```python
from build123d import *

# Parameters (mm, degrees)
BOSS_EXTRUDE1_DEPTH = 1.445
SKETCH2_R           = 3.2
CUT_EXTRUDE1_DEPTH  = 1.67
SKETCH3_R           = 3.2
BOSS_EXTRUDE2_DEPTH = 3.4
CUT_EXTRUDE3_DEPTH  = 36.101138158
SKETCH6_R           = 1.65
CUT_EXTRUDE4_DEPTH  = 34.904858059
BOSS_EXTRUDE3_DEPTH = 2.89
BOSS_EXTRUDE4_DEPTH = 31
BOSS_EXTRUDE5_DEPTH = 2.75
FILLET2_R           = 1


with BuildPart() as part:
    # Sketch1 → Boss-Extrude1 (new, symmetric)
    with BuildSketch(Plane.XY):
        with BuildLine():
            Line((4.65938028, -4.314241), (22.15938028, 14.585759))
            ThreePointArc((22.15938028, 14.585759), (21.814241, 23.55938028), (12.84061972, 23.214241))
            Line((12.84061972, 23.214241), (-4.65938028, 4.314241))
            ThreePointArc((-4.65938028, 4.314241), (-4.314241, -4.65938028), (4.65938028, -4.314241))
        make_face()
    extrude(amount=BOSS_EXTRUDE1_DEPTH, both=True)

    # Sketch2 → Cut-Extrude1 (cut)
    with BuildSketch(Plane.XY.offset(1.445)):
        Circle(SKETCH2_R)
        with Locations((17.5, 18.9)):
            Circle(SKETCH2_R)
    extrude(amount=-CUT_EXTRUDE1_DEPTH, mode=Mode.SUBTRACT)

    # Sketch3 → Boss-Extrude2 (add)
    with BuildSketch(Plane.XY.offset(-0.225)):
        Circle(SKETCH3_R)
        with Locations((17.5, 18.9)):
            Circle(SKETCH3_R)
    extrude(amount=-BOSS_EXTRUDE2_DEPTH)

    # Sketch5 → Cut-Extrude3 (cut, through all)
    with BuildSketch(Plane.XY.offset(1.445)):
        with BuildLine():
            Line((22.37, 14.825003067), (22.37, 22.974996933))
            ThreePointArc((22.37, 22.974996933), (23.85, 18.9), (22.37, 14.825003067))
        make_face()
    extrude(amount=-CUT_EXTRUDE3_DEPTH, mode=Mode.SUBTRACT)

    # Sketch6 → Cut-Extrude4 (cut, through all)
    with BuildSketch(Plane.XY.offset(-0.225)):
        Circle(SKETCH6_R)
        with Locations((17.5, 18.9)):
            Circle(SKETCH6_R)
    extrude(amount=-CUT_EXTRUDE4_DEPTH, mode=Mode.SUBTRACT)

    # Sketch7 → Boss-Extrude3 (add)
    with BuildSketch(Plane.XY.offset(1.445)):
        with BuildLine():
            Line((-4.65938028, 4.314241), (-13, 4.314241))
            Line((-13, 4.314241), (-13, -6.35))
            Line((-13, -6.35), (0, -6.35))
            ThreePointArc((0, -6.35), (-5.818845691, -2.542348289), (-4.65938028, 4.314241))
        make_face()
    extrude(amount=-BOSS_EXTRUDE3_DEPTH)

    # Sketch8 → Boss-Extrude4 (add)
    with BuildSketch(Plane.XZ.offset(6.35)):
        with BuildLine():
            Line((-13.837814719, 2.538922528), (-13, 1.445))
            Line((-13, 1.445), (-10.25, 1.445))
            Line((-10.25, 1.445), (-10.25, 3.755))
            ThreePointArc((-10.25, 3.755), (-12.892016574, 5.649152771), (-13.837814719, 2.538922528))
        make_face()
        Polygon((-11.25, 3.177649731), (-12.25, 2.600299462), (-13.25, 3.177649731), (-13.25, 4.332350269), (-12.25, 4.909700538), (-11.25, 4.332350269), align=None, mode=Mode.SUBTRACT)
    extrude(amount=-BOSS_EXTRUDE4_DEPTH)

    # Sketch10 → Boss-Extrude5 (add)
    with BuildSketch(Plane.ZY.offset(13)):
        Polygon((-1.445, 4.314241), (1.445, 24.65), (1.445, 4.314241), align=None)
    extrude(amount=-BOSS_EXTRUDE5_DEPTH)

    # Fillet2
    fillet2_edges = [part.edges().sort_by_distance(p)[0] for p in [
        (-4.65938028, 4.314241, 0),
        (-11.625, 24.65, 1.445),
    ]]
    fillet(fillet2_edges, radius=FILLET2_R)


solid = part.part
```
Can you work these out from the model? Positions are in its coordinate system, mm. A direction names the side the tool comes from. Give positions to 0.01 mm unless a question says otherwise; leave off trailing zeros. Order: outer loops, then holes, each group sorted by start corner. A loop starts at its lowest first (then second) coordinate and runs counter-clockwise, first axis right, second up. Notation, with made-up numbers: (70, 87.5) - (117, 87.5) arc R34 ccw to (117, 123.5) - close; hole circle Ø8 at (75, 42.25). An arc over 180 degrees is marked (long way). Use a Markdown table: item, result. Add a question column.
Q1. I'm going to push flat-ended pins straight in: pin 1 (16 mm diameter, centred on x = 2, y = 11.5, fed in from -Z) (3 decimals); pin 2 (4 mm diameter, centred on x = 16, z = 1, fed in from -Y); pin 3 (1 mm diameter, centred on x = 13.5, y = 14, fed in from +Z) (3 decimals). Where does each tip first touch, or does it pass through?
Q2. On a 3-axis mill with a long thin cutter (end or side, diameter ignored), from which of +Z, -Z, +X, -X, +Y, -Y can I reach the whole of each face in a straight line? I mean faces 1 (the flat face through (-11.743, 8.933, 2.893)), 2 (the cylindrical face through (-11.55, 24.4, 1.65)), 3 (the flat face through (-8, 4.314, 0)), 4 (the cylindrical face through (16.806, 15.776, 0.622)), 5 (the flat face through (-10.25, 9, 2)). Say none if no direction works.
Q3. Please list where these lines run through material, in increasing order: line 1 along Y through (x, z) = (0, -3); line 2 along Y through (x, z) = (-9, 0); line 3 along Z through (x, y) = (15.5, 17) (3 decimals).
Q4. If we section it at A-A on y = 18.9: Write out the boundary of the cut face in (x, z) (3 decimals).
Q5. If we section it at B-B on x = 17.5: Write out the boundary of the cut face in (y, z) (3 decimals).
Q6. If we section it at C-C on y = 0: Write out the boundary of the cut face in (x, z) (3 decimals).
Q7. If we mould it in two halves opening along X, with no side actions, what happens to faces 6 (the flat face through (6, 6, 1.445)), 7 (the cylindrical face through (-12.841, 8.933, 5.666)), 8 (the flat face through (-13, 6, 0)), 9 (the flat face through (-13.25, 9, 4))? For each: released by +X, released by -X, zero draft, split by the parting line, or undercut.
Q8. If we section it at D-D on z = 0.75: Write out the boundary of the cut face in (x, y) (3 decimals), plus the area to 3 significant figures.
Answers follow:
| question | item | result |
|---|---|---|
| 1 | pin 1 | stops at z = -1.445 |
| 1 | pin 2 | stops at y = 5.77 |
| 1 | pin 3 | stops at z = 1.445 |
| 2 | face 1 | +Y, -Y |
| 2 | face 2 | -Z, -X, +Y |
| 2 | face 3 | +Z, -Z, +Y |
| 2 | face 4 | +Z |
| 2 | face 5 | +Z, +Y |
| 3 | line 1 | y = -3.2 to -1.65, 1.65 to 3.2 |
| 3 | line 2 | y = -6.35 to 4.31 |
| 3 | line 3 | z = -3.625 to -0.225 |
| 4 | outline | (-13.838, 2.539) - (-13, 1.445) - (-13, 0.628) - (-10.25, 0.628) - (-10.25, 3.755) arc R2 ccw (long way) to start; (8.846, -1.445) - (14.3, -1.445) - (14.3, -3.625) - (15.85, -3.625) - (15.85, -0.225) - (14.3, -0.225) - (14.3, 1.445) - (8.846, 1.445) - close; (19.15, -3.625) - (20.7, -3.625) - (20.7, -1.445) - (22.37, -1.445) - (22.37, 1.445) - (20.7, 1.445) - (20.7, -0.225) - (19.15, -0.225) - close; hole (-13.25, 3.178) - (-12.25, 2.6) - (-11.25, 3.178) - (-11.25, 4.332) - (-12.25, 4.91) - (-13.25, 4.332) - close |
| 5 | outline | (9.554, -1.445) - (15.7, -1.445) - (15.7, -3.625) - (17.25, -3.625) - (17.25, -0.225) - (15.7, -0.225) - (15.7, 1.445) - (9.554, 1.445) - close; (20.55, -3.625) - (22.1, -3.625) - (22.1, -1.445) - (25.25, -1.445) - (25.25, 1.445) - (22.1, 1.445) - (22.1, -0.225) - (20.55, -0.225) - close |
| 6 | outline | (-13.838, 2.539) - (-13, 1.445) - (-13, -1.445) - (-3.2, -1.445) - (-3.2, -3.625) - (-1.65, -3.625) - (-1.65, -0.225) - (-3.2, -0.225) - (-3.2, 1.445) - (-10.25, 1.445) - (-10.25, 3.755) arc R2 ccw (long way) to start; (1.65, -3.625) - (3.2, -3.625) - (3.2, -1.445) - (8.654, -1.445) - (8.654, 1.445) - (3.2, 1.445) - (3.2, -0.225) - (1.65, -0.225) - close; hole (-13.25, 3.178) - (-12.25, 2.6) - (-11.25, 3.178) - (-11.25, 4.332) - (-12.25, 4.91) - (-13.25, 4.332) - close |
| 7 | face 6 | zero draft |
| 7 | face 7 | split by the parting line |
| 7 | face 8 | released by -X |
| 7 | face 9 | undercut |
| 8 | outline | (-13, -6.35) - (0, -6.35) arc R6.35 ccw to (4.659, -4.314) - (22.159, 14.586) arc R6.35 ccw to (22.37, 14.825) - (22.37, 22.975) arc R6.35 ccw to (12.841, 23.214) - (-4.363, 4.635) arc R1 cw to (-5.096, 4.314) - (-10.25, 4.314) - (-10.25, 19.76) - (-13, 19.76) - close; hole circle Ø6.4 at (0, 0); hole circle Ø6.4 at (17.5, 18.9) |
| 8 | area | 506 mm^2 |
